Model file for the job. Use its own axes, mm. A direction names the side the tool comes from. Give positions to 0.01 mm unless a question says otherwise; leave off trailing zeros. Loops run counter-clockwise (first coordinate to the right, second up) from the corner with the lowest first, then second, coordinate; pieces in that order, holes last. Notation, with made-up numbers: M 39,84 L 98,84 A16 ccw 98,115 Z; hole C 52,82 d1. An arc over 180 degrees is marked long. Answer in a Markdown table with one row per item.
```python
from build123d import *

# Parameters (mm, degrees)
SKETCH1_W                     = 13.843
SKETCH1_H                     = 13.843
MAIN_BODY_EXTRUDE_DEPTH       = 10.16
MAIN_BODY_CUT_DEPTH           = 9.36
SKETCH21_R                    = 0.635
SCREW_HOLES_CUT_DEPTH         = 23.056357315
X_AXIS_SLOT_DEPTH             = 23.056357315
SKETCH6_W                     = 5.08
SKETCH6_H                     = 6.485700116
Y_AXIS_SLOT_DEPTH             = 23.056357315
SPRING_START                  = 0.8
SKETCH11_W                    = 11.303
SKETCH11_H                    = 11.303
SKETCH11_R                    = 4.826
SKETCH11_R_2                  = 0.635
SPRING_RETAINER_EXTRUDE_DEPTH = 0.8
SKETCH12_R                    = 2.54
STICK_SUPPORT_DEPTH           = 5.3595
SKETCH20_R                    = 2.54
BOSS_EXTRUDE9_DEPTH           = 2.54
FILLET4_R                     = 2.54


with BuildPart() as part:
    # Sketch1 → main body extrude (new body)
    with BuildSketch(Plane(origin=(0, 0, 0), x_dir=(1, 0, 0), z_dir=(0, 1, 0))):
        with Locations((6.9215, 6.9215)):
            Rectangle(SKETCH1_W, SKETCH1_H)
    extrude(amount=MAIN_BODY_EXTRUDE_DEPTH)

    # Sketch4 → main body cut (cut)
    with BuildSketch(Plane(origin=(0, 10.16, 0), x_dir=(1, 0, 0), z_dir=(0, 1, 0))):
        with BuildLine():
            Line((1.735593231, 10.498593231), (1.27, 10.033))
            Line((1.27, 10.033), (1.27, 3.81))
            Line((1.27, 3.81), (1.735593231, 3.344406769))
            ThreePointArc((1.735593231, 3.344406769), (2.868191287, 2.999925058), (3.3565, 1.9215))
            ThreePointArc((3.3565, 1.9215), (3.353473501, 1.828350157), (3.344406769, 1.735593231))
            Line((3.344406769, 1.735593231), (3.81, 1.27))
            Line((3.81, 1.27), (10.033, 1.27))
            Line((10.033, 1.27), (10.498593231, 1.735593231))
            ThreePointArc((10.498593231, 1.735593231), (10.906801769, 2.936198231), (12.107406769, 3.344406769))
            Line((12.107406769, 3.344406769), (12.573, 3.81))
            Line((12.573, 3.81), (12.573, 10.033))
            Line((12.573, 10.033), (12.107406769, 10.498593231))
            ThreePointArc((12.107406769, 10.498593231), (10.906801769, 10.906801769), (10.498593231, 12.107406769))
            Line((10.498593231, 12.107406769), (10.033, 12.573))
            Line((10.033, 12.573), (3.81, 12.573))
            Line((3.81, 12.573), (3.344406769, 12.107406769))
            ThreePointArc((3.344406769, 12.107406769), (3.353473501, 12.014649843), (3.3565, 11.9215))
            ThreePointArc((3.3565, 11.9215), (2.868191287, 10.843074942), (1.735593231, 10.498593231))
        make_face()
    extrude(amount=-MAIN_BODY_CUT_DEPTH, mode=Mode.SUBTRACT)

    # Sketch21 → screw holes cut (cut, through all)
    with BuildSketch(Plane(origin=(0, 10.16, 0), x_dir=(1, 0, 0), z_dir=(0, 1, 0))):
        with Locations(Location((1.9215, 11.9215, 0), (0, 0, 270))):
            Circle(SKETCH21_R)
        with Locations(Location((11.9215, 11.9215, 0), (0, 0, 270))):
            Circle(SKETCH21_R)
        with Locations(Location((11.9215, 1.9215, 0), (0, 0, 270))):
            Circle(SKETCH21_R)
        with Locations(Location((1.9215, 1.9215, 0), (0, 0, 270))):
            Circle(SKETCH21_R)
    extrude(amount=-SCREW_HOLES_CUT_DEPTH, mode=Mode.SUBTRACT)

    # Sketch5 → x axis slot (cut, through all)
    with BuildSketch(Plane.XY):
        with BuildLine():
            Line((9.4615, 12.711621125), (4.3815, 12.711621125))
            Line((4.3815, 12.711621125), (4.3815, 6.1595))
            Line((4.3815, 6.1595), (5.6515, 6.1595))
            ThreePointArc((5.6515, 6.1595), (6.9215, 4.8895), (8.1915, 6.1595))
            Line((8.1915, 6.1595), (9.4615, 6.1595))
            Line((9.4615, 6.1595), (9.4615, 12.711621125))
        make_face()
    extrude(amount=-X_AXIS_SLOT_DEPTH, mode=Mode.SUBTRACT)

    # Sketch6 → y axis slot (cut, through all)
    with BuildSketch(Plane(origin=(13.843, 0, 0), x_dir=(0, 0, -1), z_dir=(1, 0, 0))):
        with BuildLine():
            Line((5.6515, 6.1595), (5.6515, 12.645200116))
            ThreePointArc((5.6515, 12.645200116), (6.9215, 13.915200116), (8.1915, 12.645200116))
            Line((8.1915, 12.645200116), (8.1915, 6.1595))
            ThreePointArc((8.1915, 6.1595), (6.9215, 4.8895), (5.6515, 6.1595))
        make_face()
        with Locations((6.9215, 9.402350058)):
            Rectangle(SKETCH6_W, SKETCH6_H)
    extrude(amount=-Y_AXIS_SLOT_DEPTH, mode=Mode.SUBTRACT)

    # Sketch11 → spring retainer extrude (add)
    with BuildSketch(Plane(origin=(0, 0.8, 0), x_dir=(1, 0, 0), z_dir=(0, 1, 0)).offset(SPRING_START)):
        with Locations((6.9215, 6.9215)):
            Rectangle(SKETCH11_W, SKETCH11_H)
        with Locations(Location((6.9215, 6.9215, 0), (0, 0, 270))):
            Circle(SKETCH11_R, mode=Mode.SUBTRACT)
        with Locations(Location((1.9215, 11.9215, 0), (0, 0, 270))):
            Circle(SKETCH11_R_2, mode=Mode.SUBTRACT)
        with Locations(Location((11.9215, 11.9215, 0), (0, 0, 270))):
            Circle(SKETCH11_R_2, mode=Mode.SUBTRACT)
        with Locations(Location((11.9215, 1.9215, 0), (0, 0, 270))):
            Circle(SKETCH11_R_2, mode=Mode.SUBTRACT)
        with Locations(Location((1.9215, 1.9215, 0), (0, 0, 270))):
            Circle(SKETCH11_R_2, mode=Mode.SUBTRACT)
    extrude(amount=-SPRING_RETAINER_EXTRUDE_DEPTH)

    # Sketch12 → Stick support (add)
    with BuildSketch(Plane(origin=(0, 0.8, 0), x_dir=(1, 0, 0), z_dir=(0, 1, 0))):
        with Locations(Location((6.9215, 6.9215, 0), (0, 0, 90))):
            Circle(SKETCH12_R)
    extrude(amount=STICK_SUPPORT_DEPTH)

    # Sketch20 → Boss-Extrude9 (add)
    with BuildSketch(Plane(origin=(0, 6.1595, 0), x_dir=(1, 0, 0), z_dir=(0, 1, 0))):
        with Locations(Location((6.9215, 6.9215, 0), (0, 0, 90))):
            Circle(SKETCH20_R)
    extrude(amount=BOSS_EXTRUDE9_DEPTH)

    # Fillet4
    fillet4_edges = [part.edges().sort_by_distance(p)[0] for p in [
        (6.9215, 8.6995, -4.3815),
    ]]
    fillet(fillet4_edges, radius=FILLET4_R)


solid = part.part
```
(1) Which spindle directions (+Z, -Z, +X, -X, +Y, -Y) get a long thin tool onto all of the face, cutting with end or side? Do faces 5 (the flat face through (12.573, 4, -7)), 6 (the flat face through (9, 6.16, -13)), 7 (the flat face through (1, 6.159, -5)). Say none if no direction does.
Established:
| item | result |
|---|---|
| face 5 | +Y |
| face 6 | -Z, +Y |
| face 7 | -X, +Y |
(2) Saw through at B-B, the plane z = -1.5. Give the cut face in (x, y), and give its area (3 significant figures).
Established:
| item | result |
|---|---|
| outline | M 0,0 L 1.45,0 L 1.45,10.16 L 0,10.16 Z; M 2.4,0 L 11.45,0 L 11.45,10.16 L 10.26,10.16 L 10.26,1.6 L 3.58,1.6 L 3.58,10.16 L 2.4,10.16 Z; M 12.4,0 L 13.84,0 L 13.84,10.16 L 12.4,10.16 Z |
| area | 64.1 mm2 |
(3) Saw through at C-C, the plane z = -6.25. Give the cut face in (x, y), and give its area (3 significant figures).
Established:
| item | result |
|---|---|
| outline | M 0,0 L 13.84,0 L 13.84,5.08 L 12.57,5.08 L 12.57,1.6 L 11.7,1.6 L 11.7,0.8 L 9.37,0.8 L 9.37,6.16 A2.45 ccw 4.47,6.16 L 4.47,0.8 L 2.14,0.8 L 2.14,1.6 L 1.27,1.6 L 1.27,5.08 L 0,5.08 Z |
| area | 59.0 mm2 |
(4) Saw through at D-D, the plane y = 9.25. Count the separate pieces of the cut face and the enclosed holes in it, and give its area (3 significant figures).
Established:
| item | result |
|---|---|
| separate pieces | 4 |
| enclosed holes | 4 |
| area | 49.5 mm2 |
(5) Wall check: L1, parallel to Z at x = 12, y = 6.5; L2, parallel to X at y = 6, z = -9.5; L3, parallel to Z at x = 10, y = 5. Give the ranges that are in metal, low to high.
Established:
| item | result |
|---|---|
| L1 | z = -13.84 to -12.55, -11.29 to -10.49, -3.35 to -2.55, -1.29 to 0 |
| L2 | x = 0 to 1.27, 12.57 to 13.84 |
| L3 | z = -13.84 to -12.57, -1.27 to 0 |
(6) Saw through at A-A, the plane y = 2. Give the cut face in (x, z) (1 decimal).
Established:
| item | result |
|---|---|
| outline | M 0,-13.8 L 13.8,-13.8 L 13.8,0 L 0,0 Z; C 6.9,-6.9 d5.1; hole C 1.9,-11.9 d1.3; hole M 1.3,-10 L 1.7,-10.5 A1.4 cw 3.3,-12.1 L 3.8,-12.6 L 10,-12.6 L 10.5,-12.1 A1.4 cw 12.1,-10.5 L 12.6,-10 L 12.6,-3.8 L 12.1,-3.3 A1.4 cw 10.5,-1.7 L 10,-1.3 L 3.8,-1.3 L 3.3,-1.7 A1.4 cw 1.7,-3.3 L 1.3,-3.8 Z; hole C 1.9,-1.9 d1.3; hole C 11.9,-11.9 d1.3; hole C 11.9,-1.9 d1.3 |
(7) Mould opens along Z. For faces 1 (the flat face through (5, 6.16, -1)), 2 (the flat face through (7, 4, 0)), 3 (the flat face through (1, 8, -9.462)), 4 (the flat face through (1, 8, -4.382)) say: pulls with the +Z half, pulls with the -Z half, needs draft (parallel to the pull), parting line crosses it, or undercut.
Established:
| item | result |
|---|---|
| face 1 | needs draft |
| face 2 | pulls with the +Z half |
| face 3 | undercut |
| face 4 | undercut |
(8) Flat gauge pins, fed straight in: P1, Ø0.6, axis at x = 13, z = -9, coming from the +Y side; P2, Ø1, axis at x = 1.92, z = -11.92, coming from the -Y side. Where does each tip first touch, or does it go through?
Established:
| item | result |
|---|---|
| P1 | stops at y = 6.16 |
| P2 | passes through |
